Build history of the part. All positions in model axes, mm. Give positions to 0.01 mm unless a question says otherwise; leave off trailing zeros. Order: outer loops, then holes, each group sorted by start corner. A loop starts at its lowest first (then second) coordinate and runs counter-clockwise, first axis right, second up. Notation, with made-up numbers: M -4,52.5 L 19,52.5 A26 cw 19,70.5 Z; hole C -7.75,-8.75 d4. An arc over 180 degrees is marked long. Use CSV: the item, a comma, the result in double quotes. Start each with the question number.
Item 1: Band-saw the part on B-B on x = 0. Write the cut outline in (y, z), plus the area to 3 significant figures.
Item 2: Band-saw the part on D-D on y = 1.25. Write the cut outline in (x, z), plus the area to 3 significant figures.
Item 3: Wall check: line 1 along X through (y, z) = (1.3, 0); line 2 along Z through (x, y) = (-17.5, 1.3); line 3 along X through (y, z) = (0.4, -1). Give the ranges that are in metal, low to high.
Item 4: Two-plate mould, pull along X, no slides. Class faces 1 (the cylindrical face through (-12.8, 1, 19.4)), 2 (the flat face through (-18, 2, 0)), 3 (the cylindrical face through (-27.334, 0.986, -6.07)): pulls with the +X half, pulls with the -X half, needs draft (parallel to the pull), parting line crosses it, or undercut.
Item 5: Pin check, flat tip, straight feed: P1, Ø1, axis at x = 7.5, y = 0, coming from the +Z side. Stop position of the tip, or through.
Item 6: Band-saw the part on C-C on x = 10.5. Write the cut outline in (y, z), plus the area to 3 significant figures.
Item 7: Band-saw the part on A-A on z = 0. Write the cut outline in (x, y), plus the area to 3 significant figures.
from build123d import *

# Parameters (mm, degrees)
SKETCH_1_R               = 28
SKETCH_1_R_2             = 2.6
EXTRUDE_1_DEPTH          = 2
CUT_EXTRUDE_2_DEPTH      = 40.648455203
CUT_EXTRUDE_2_DEPTH_BACK = 40.648455203


with BuildPart() as part:
    # 草图1 → 凸台-拉伸1 (new body)
    with BuildSketch(Plane(origin=(0, 0, 0), x_dir=(1, 0, 0), z_dir=(0, 1, 0))):
        with Locations(Location((0, 0, 0), (0, 0, 270))):
            Circle(SKETCH_1_R)
        with Locations(Location((10.5, 18.186533479, 0), (0, 0, 270))):
            Circle(SKETCH_1_R_2, mode=Mode.SUBTRACT)
        with Locations(Location((21, 0, 0), (0, 0, 270))):
            Circle(SKETCH_1_R_2, mode=Mode.SUBTRACT)
        with Locations(Location((10.5, -18.186533479, 0), (0, 0, 270))):
            Circle(SKETCH_1_R_2, mode=Mode.SUBTRACT)
        with Locations(Location((-10.5, -18.186533479, 0), (0, 0, 270))):
            Circle(SKETCH_1_R_2, mode=Mode.SUBTRACT)
        with Locations(Location((-21, 0, 0), (0, 0, 270))):
            Circle(SKETCH_1_R_2, mode=Mode.SUBTRACT)
        with Locations(Location((-10.5, 18.186533479, 0), (0, 0, 270))):
            Circle(SKETCH_1_R_2, mode=Mode.SUBTRACT)
    extrude(amount=EXTRUDE_1_DEPTH)

    # 草图4 → 切除-拉伸2 (cut, two sides: drawn at the far end of the back side and taken through both)
    with BuildSketch(Plane(origin=(0, 2, 0), x_dir=(1, 0, 0), z_dir=(0, 1, 0)).offset(-CUT_EXTRUDE_2_DEPTH_BACK)):
        with BuildLine():
            ThreePointArc((4.758569662, 16.444127766), (7.4999998, 12.990381172), (11.861747108, 12.343105991))
            ThreePointArc((11.861747108, 12.343105991), (17.29701741, 9.986437924), (16.620317219, 4.10102167))
            ThreePointArc((16.620317219, 4.10102167), (15, 2.31e-07), (16.620316904, -4.101021333))
            ThreePointArc((16.620316904, -4.101021333), (17.297017641, -9.986437525), (11.861747557, -12.343106096))
            ThreePointArc((11.861747557, -12.343106096), (7.5000002, -12.990380941), (4.758569796, -16.444127324))
            ThreePointArc((4.758569796, -16.444127324), (2.31e-07, -19.972875449), (-4.758569662, -16.444127766))
            ThreePointArc((-4.758569662, -16.444127766), (-7.4999998, -12.990381172), (-11.861747108, -12.343105991))
            ThreePointArc((-11.861747108, -12.343105991), (-17.29701741, -9.986437924), (-16.620317219, -4.10102167))
            ThreePointArc((-16.620317219, -4.10102167), (-15, -2.31e-07), (-16.620316904, 4.101021333))
            ThreePointArc((-16.620316904, 4.101021333), (-17.297017641, 9.986437525), (-11.861747557, 12.343106096))
            ThreePointArc((-11.861747557, 12.343106096), (-7.5000002, 12.990380941), (-4.758569796, 16.444127324))
            ThreePointArc((-4.758569796, 16.444127324), (-2.31e-07, 19.972875449), (4.758569662, 16.444127766))
        make_face()
    extrude(amount=CUT_EXTRUDE_2_DEPTH + CUT_EXTRUDE_2_DEPTH_BACK, mode=Mode.SUBTRACT)


solid = part.part
Model answer:
1,outline,"M 0,-28 L 2,-28 L 2,-19.97 L 0,-19.97 Z; M 0,19.97 L 2,19.97 L 2,28 L 0,28 Z"
1,area,"32.1 mm^2"
2,outline,"C 0,0 d56; hole C -21,0 d5.2; hole M -16.62,-4.1 A4.97 ccw -11.86,-12.34 A6 cw -4.76,-16.44 A4.97 ccw 4.76,-16.44 A6 cw 11.86,-12.34 A4.97 ccw 16.62,-4.1 A6 cw 16.62,4.1 A4.97 ccw 11.86,12.34 A6 cw 4.76,16.44 A4.97 ccw -4.76,16.44 A6 cw -11.86,12.34 A4.97 ccw -16.62,4.1 A6 cw Z; hole C -10.5,-18.19 d5.2; hole C -10.5,18.19 d5.2; hole C 10.5,-18.19 d5.2; hole C 10.5,18.19 d5.2; hole C 21,0 d5.2"
2,area,"1,360 mm^2"
3,line 1,"x = -28 to -23.6, -18.4 to -15, 15 to 18.4, 23.6 to 28"
3,line 2,"z = -21.86 to -9.6, -5.4 to 5.4, 9.6 to 21.86"
3,line 3,"x = -27.98 to -23.4, -18.6 to -15.08, 15.08 to 18.6, 23.4 to 27.98"
4,face 1,"undercut"
4,face 2,"needs draft"
4,face 3,"parting line crosses it"
5,P1,"stops at z = 27.11"
6,outline,"M 0,-25.96 L 2,-25.96 L 2,-20.79 L 0,-20.79 Z; M 0,-15.59 L 2,-15.59 L 2,-12.19 L 0,-12.19 Z; M 0,12.19 L 2,12.19 L 2,15.59 L 0,15.59 Z; M 0,20.79 L 2,20.79 L 2,25.96 L 0,25.96 Z"
6,area,"34.3 mm^2"
7,outline,"M -28,0 L -23.6,0 L -23.6,2 L -28,2 Z; M -18.4,0 L -15,0 L -15,2 L -18.4,2 Z; M 15,0 L 18.4,0 L 18.4,2 L 15,2 Z; M 23.6,0 L 28,0 L 28,2 L 23.6,2 Z"
7,area,"31.2 mm^2"
